Build history of the part. All positions in model axes, mm. A direction names the side the tool comes from. Give positions to 0.01 mm unless a question says otherwise; leave off trailing zeros. Write each loop counter-clockwise with the first axis right and the second up, starting at its lowest first coordinate (ties: lowest second). Pieces come first, ordered by that corner, then holes. Notation, with made-up numbers: (51, 51.25) -> (58, 51.25) arc R21 cw to (58, 76.25) -> close; hole circle Ø8 at (58.5, 87). An arc over 180 degrees is marked (long way). Put each result on its own line as item: value.
from build123d import *

# Parameters (mm, degrees)
BOSS_EXTRUDE1_DEPTH = 9
CUT_EXTRUDE1_DEPTH  = 7
CUT_EXTRUDE2_DEPTH  = 2.6
BOSS_EXTRUDE2_DEPTH = 3


with BuildPart() as part:
    # Sketch1 → Boss-Extrude1 (new, symmetric)
    with BuildSketch(Plane.XY):
        Polygon((0, 0), (0, 18), (3, 18), (18, 3), (18, 0), align=None)
    extrude(amount=BOSS_EXTRUDE1_DEPTH, both=True)

    # Sketch2 → Cut-Extrude1 (cut, symmetric)
    with BuildSketch(Plane.XY):
        Polygon((3, 18), (3, 3), (18, 3), align=None)
    extrude(amount=CUT_EXTRUDE1_DEPTH, both=True, mode=Mode.SUBTRACT)

    # Sketch3 → Cut-Extrude2 (cut, symmetric)
    with BuildSketch(Plane.XY):
        Polygon((0, 14), (3, 14), (3, 7), (0, 4), align=None)
        Polygon((7, 3), (14, 3), (14, 0), (4, 0), align=None)
    extrude(amount=CUT_EXTRUDE2_DEPTH, both=True, mode=Mode.SUBTRACT)

    # Sketch4 → Boss-Extrude2 (add, symmetric)
    with BuildSketch(Plane.XY):
        Polygon((1.504575227, -1.8), (0.511249685, -0.790946088), (1.234750477, 0), (3.535533906, 0), align=None)
        Polygon((0, 3.535533906), (-1.8, 1.504575227), (-0.790946088, 0.511249685), (0, 1.234750477), align=None)
        Polygon((0, 17.3), (0, 14.999216572), (-0.790946088, 14.275715779), (-1.8, 15.269041321), align=None)
        Polygon((14.999216572, 0), (14.275715779, -0.790946088), (15.269041321, -1.8), (17.3, 0), align=None)
    extrude(amount=BOSS_EXTRUDE2_DEPTH, both=True)


solid = part.part
1) Slice it at A-A (x = 8). Write the cut outline in (y, z).
Filled sheet:
outline: (0, -9) -> (13, -9) -> (13, -7) -> (3, -7) -> (3, -2.6) -> (0, -2.6) -> close; (0, 2.6) -> (3, 2.6) -> (3, 7) -> (13, 7) -> (13, 9) -> (0, 9) -> close
2) Slice it at B-B (y = 10.75). Write the cut outline in (x, z), plus the area to 3 significant figures.
Filled sheet:
outline: (0, -9) -> (10.25, -9) -> (10.25, -7) -> (3, -7) -> (3, -2.6) -> (0, -2.6) -> close; (0, 2.6) -> (3, 2.6) -> (3, 7) -> (10.25, 7) -> (10.25, 9) -> (0, 9) -> close
area: 67.4 mm2
3) Slice it at D-D (y = 6). Write the cut outline in (x, z).
Filled sheet:
outline: (0, -9) -> (15, -9) -> (15, -7) -> (3, -7) -> (3, 7) -> (15, 7) -> (15, 9) -> (0, 9) -> (0, 2.6) -> (2, 2.6) -> (2, -2.6) -> (0, -2.6) -> close
4) Wall check: L1, parallel to Z at x = 6.5, y = 13.75; L2, parallel to Y at x = 11.5, z = -3; L3, parallel to X at y = 0.75, z = 3.75. Give the ranges that are in metal, low to high.
Filled sheet:
L1: -9 to -7, 7 to 9
L2: 0 to 3
L3: 0 to 18
5) Pin check, flat tips, straight feed: pin 1 (3 mm diameter, centred on x = 10, z = -7, fed in from -Y); pin 2 (4 mm diameter, centred on x = 7, z = -5.5, fed in from +Y); pin 3 (0.5 mm diameter, centred on x = -1, y = 2.5, fed in from +Z). Stop position of each tip, or through.
Filled sheet:
pin 1: y = 0
pin 2: y = 15.32
pin 3: z = 3
6) Pull direction Y, two halves, no side cores. Call faces 5 (the flat face through (-1.3, 1.01, -0.04)), 6 (the flat face through (2, 10, 2.6)), 7 (the flat face through (15, -1, 3)): released by +Y, released by -Y, zero draft, split by the parting line, or undercut.
Filled sheet:
face 5: released by -Y
face 6: undercut
face 7: zero draft
7) Tool access for faces 1 (the flat face through (2, 6, 0)), 2 (the flat face through (14, 2, 0)), 3 (the flat face through (10, 3, 3)), 4 (the flat face through (-1, 15, 3)): list every direction of +Z, -Z, +X, -X, +Y, -Y with a clear straight run to the whole face (end or side of a thin tool).
Filled sheet:
face 1: -X
face 2: +Y, -Y
face 3: +X, +Y
face 4: +Z, -X, +Y, -Y
8) Slice it at C-C (z = -6). Write the cut outline in (x, y), plus the area to 3 significant figures.
Filled sheet:
outline: (0, 0) -> (18, 0) -> (18, 3) -> (3, 3) -> (3, 18) -> (0, 18) -> close
area: 99.0 mm2
